from build123d import *

# Parameters (mm, degrees)
BOSS_EXTRUDE1_DEPTH = 8
SKETCH2_W           = 4
SKETCH2_H           = 4
CUT_EXTRUDE1_DEPTH  = 4
CUT_EXTRUDE2_DEPTH  = 2
BOSS_EXTRUDE2_DEPTH = 6
CUT_EXTRUDE4_DEPTH  = 2
CUT_EXTRUDE5_DEPTH  = 3
CUT_EXTRUDE8_DEPTH  = 1
CUT_EXTRUDE9_DEPTH  = 1


with BuildPart() as part:
    # Sketch1 → Boss-Extrude1 (new body)
    with BuildSketch(Plane.XY):
        with BuildLine():
            Line((0, 0), (-3, 0))
            Line((-3, 0), (-5, 0))
            Line((-5, 0), (-5, 2))
            Line((-5, 2), (-2.6, 5.2))
            ThreePointArc((-2.6, 5.2), (-1.894427191, 5.788854382), (-1, 6))
            Line((-1, 6), (0, 6))
            Line((0, 6), (0, 0))
        make_face()
    extrude(amount=BOSS_EXTRUDE1_DEPTH)

    # Sketch2 → Cut-Extrude1 (cut)
    with BuildSketch(Plane(origin=(0, 6, 0), x_dir=(1, 0, 0), z_dir=(0, 1, 0))):
        with Locations((-3, -4)):
            Rectangle(SKETCH2_W, SKETCH2_H)
    extrude(amount=-CUT_EXTRUDE1_DEPTH, mode=Mode.SUBTRACT)

    # Sketch3 → Cut-Extrude2 (cut, through all)
    with BuildSketch(Plane.ZY.offset(1)):
        with BuildLine():
            Line((3, 6), (3, 5))
            ThreePointArc((3, 5), (4, 4), (5, 5))
            Line((5, 5), (5, 6))
            Line((5, 6), (3, 6))
        make_face()
    extrude(amount=-CUT_EXTRUDE2_DEPTH, mode=Mode.SUBTRACT)

    # Sketch5 → Boss-Extrude2 (add)
    with BuildSketch(Plane.XY.offset(8)):
        with BuildLine():
            Line((-5, 0), (-7, 0))
            ThreePointArc((-7, 0), (-6.414213562, 1.414213562), (-5, 2))
            Line((-5, 2), (-5, 0))
        make_face()
    extrude(amount=-BOSS_EXTRUDE2_DEPTH)

    # Sketch6 → Cut-Extrude4 (cut)
    with BuildSketch(Plane.XY.offset(8)):
        with BuildLine():
            Line((-5, 2), (-5, 0))
            Line((-5, 0), (-7, 0))
            ThreePointArc((-7, 0), (-6.414213562, 1.414213562), (-5, 2))
        make_face()
    extrude(amount=-CUT_EXTRUDE4_DEPTH, mode=Mode.SUBTRACT)

    # Sketch7 → Cut-Extrude5 (cut, through all)
    with BuildSketch(Plane(origin=(0, 2, 0), x_dir=(1, 0, 0), z_dir=(0, 1, 0))):
        with BuildLine():
            Line((-4, -3), (-3, -3))
            ThreePointArc((-3, -3), (-2, -4), (-3, -5))
            Line((-3, -5), (-4, -5))
            ThreePointArc((-4, -5), (-5, -4), (-4, -3))
        make_face()
    extrude(amount=-CUT_EXTRUDE5_DEPTH, mode=Mode.SUBTRACT)

    # Sketch8 → Cut-Extrude8 (cut)
    with BuildSketch(Plane.XY.offset(8)):
        with BuildLine():
            Line((-5, 0), (-3, 0))
            Line((-3, 0), (-3, 4))
            ThreePointArc((-3, 4), (-2.897366596, 4.632455532), (-2.6, 5.2))
            Line((-2.6, 5.2), (-5, 2))
            Line((-5, 2), (-5, 0))
        make_face()
    extrude(amount=-CUT_EXTRUDE8_DEPTH, mode=Mode.SUBTRACT)

    # Sketch9 → Cut-Extrude9 (cut)
    with BuildSketch(Plane(origin=(0, 0, 0), x_dir=(-1, 0, 0), z_dir=(0, 0, -1))):
        with BuildLine():
            Line((5, 0), (5, 2))
            Line((5, 2), (2.6, 5.2))
            ThreePointArc((2.6, 5.2), (2.897366596, 4.632455532), (3, 4))
            Line((3, 4), (3, 0))
            Line((3, 0), (5, 0))
        make_face()
    extrude(amount=-CUT_EXTRUDE9_DEPTH, mode=Mode.SUBTRACT)


solid = part.part
The listing builds one solid part. Answer for the finished solid, in the listing's coordinates (mm). A direction names the side the tool comes from. Give positions to 0.01 mm unless a question says otherwise; leave off trailing zeros. Loops run counter-clockwise (first coordinate to the right, second up) from the corner with the lowest first, then second, coordinate; pieces in that order, holes last.
Item 1: Determine the mould class of faces 5 (the flat face through (-3, 4, 2)), 6 (the flat face through (-4, 2, 7)), 7 (the flat face through (-6, 1, 2)), 8 (the flat face through (-3, 2, 0.5)) for opening direction Z: +Z half, -Z half, draft (parallel to the pull), parting line (faces both ways), or undercut.
Derived:
face 5: undercut
face 6: +Z half
face 7: -Z half
face 8: draft
Item 2: A cutting plane is placed at C-C (x = -0.5). Give the vertices of the cut face in (y, z), then the cut area to 3 significant figures.
Derived:
outline: (0, 0) - (6, 0) - (6, 3) - (5, 3) arc R1 cw to (5, 5) - (6, 5) - (6, 8) - (0, 8) - close
area: 44.4 mm2
Item 3: A cutting plane is placed at B-B (y = 0.4). Give the vertices of the cut face in (x, z).
Derived:
outline: (-6.96, 2) - (-5, 2) - (-5, 1) - (-3, 1) - (-3, 0) - (0, 0) - (0, 8) - (-3, 8) - (-3, 7) - (-5, 7) - (-5, 6) - (-6.96, 6) - close; hole (-4, 3) - (-3, 3) arc R1 ccw to (-3, 5) - (-4, 5) arc R1 ccw to start
Item 4: A tool of negligible diameter and unlimited length cuts with its end or side. For faces 1 (the flat face through (-5, 1, 1.5)), 2 (the flat face through (-1.7, 2, 4)), 3 (the flat face through (-3, 2, 7.5)), 4 (the flat face through (-0.5, 5.5, 3)), from which of +Z, -Z, +X, -X, +Y, -Y can it reach the whole face along a straight path? Write none if from no direction.
Derived:
face 1: -Z, -X, +Y, -Y
face 2: -X, +Y
face 3: +Z, -X, +Y, -Y
face 4: +X, -X, +Y
Item 5: Find the intervals of material crossed by line 1 along Z through (x, y) = (-3.75, 3.15); line 2 along Z through (x, y) = (-1.5, 3); line 3 along X through (y, z) = (2.25, 3), in increasing order.
Derived:
line 1: z = 1 to 2, 6 to 7
line 2: z = 0 to 2, 6 to 8
line 3: x = -1 to 0
Item 6: Each of these flat-tipped pins is pushed along its axis until it touches: pin 1 Ø1 at (x, y) = (-6.5, 1.5) entering from -Z; pin 2 Ø0.8 at (x, y) = (-3.5, 0.5) entering from -Z; pin 3 Ø0.5 at (x, y) = (-3.5, 1) entering from +Z. Where does it stop, or does it pass through?
Derived:
pin 1: stops at z = 2
pin 2: stops at z = 1
pin 3: stops at z = 7
Item 7: A cutting plane is placed at A-A (z = 4.75). Give the vertices of the cut face in (x, y).
Derived:
outline: (-7, 0) - (-4.66, 0) - (-4.66, 2) - (-5, 2) arc R2 ccw to start; (-2.34, 0) - (0, 0) - (0, 4.34) - (-1, 4.34) - (-1, 2) - (-2.34, 2) - close
